from build123d import *

# Parameters (mm, degrees)
CROQUIS1_W              = 4
CROQUIS1_H              = 11
SALIENTE_EXTRUIR1_DEPTH = 100
SALIENTE_EXTRUIR2_DEPTH = 11
REDONDEO1_R             = 10


with BuildPart() as part:
    # Croquis1 → Saliente-Extruir1 (new body)
    with BuildSketch(Plane.XY):
        with Locations((-13, 0)):
            Rectangle(CROQUIS1_W, CROQUIS1_H)
    extrude(amount=-SALIENTE_EXTRUIR1_DEPTH)

    # Croquis3 → Saliente-Extruir2 (add)
    with BuildSketch(Plane.XZ.offset(5.5)):
        Polygon((-15, -100), (-30.130974356, -100), (-15, -76.782527914), align=None)
    extrude(amount=-SALIENTE_EXTRUIR2_DEPTH)

    # Redondeo1
    redondeo1_edges = [part.edges().sort_by_distance(p)[0] for p in [
        (-15, 0, -76.782527914),
    ]]
    fillet(redondeo1_edges, radius=REDONDEO1_R)


solid = part.part
Design review of the part built by this model. Coordinates are the model's own, in mm. A direction names the side the tool comes from. Give positions to 0.01 mm unless a question says otherwise; leave off trailing zeros. Order: outer loops, then holes, each group sorted by start corner. A loop starts at its lowest first (then second) coordinate and runs counter-clockwise, first axis right, second up. Notation, with made-up numbers: (77, -5) - (133, -5) arc R28 cw to (133, 27) - close; hole circle Ø11 at (7, -16). An arc over 180 degrees is marked (long way). Use CSV: the item, a comma, the result in double quotes. Start each with the question number.
Q1. Machinability: for faces 1 (the face through (-15, 0, -36)), 2 (the face through (-20, 0, -100)), which of the approach directions +Z, -Z, +X, -X, +Y, -Y give a long, thin tool a straight path to every point of the face, cutting with its end or side? Answer none if there is none.
Q2. Take a section at C-C (x = -22). State the section outline as (y, z) points, and give its area (3 significant figures).
Q3. For line 1 (X direction, y = 4, z = -39); line 2 (Z direction, x = -28.5, y = 0.5); line 3 (Z direction, x = -24.25, y = 3), list the stretches that pass through material, from the lowest coordinate up.
Q4. Take a section at A-A (y = -0.5). State the section outline as (x, z) points, and give its area (3 significant figures).
Q5. Take a section at B-B (z = -53). State the section outline as (x, y) points, and give its area (3 significant figures).
Q6. For P1, Ø3.5, axis at y = 1.5, z = -55.5, coming from the -X side, flat-tipped, find the tip position at first contact; note if it passes through.
Calculated:
1,face 1,"+Z, -X, +Y, -Y"
1,face 2,"-Z, +X, -X, +Y, -Y"
2,outline,"(-5.5, -100) - (5.5, -100) - (5.5, -87.52) - (-5.5, -87.52) - close"
2,area,"137 mm²"
3,line 1,"x = -15 to -11"
3,line 2,"z = -100 to -97.5"
3,line 3,"z = -100 to -90.98"
4,outline,"(-30.13, -100) - (-11, -100) - (-11, 0) - (-15, 0) - (-15, -73.81) arc R10 cw to (-16.62, -79.27) - close"
4,area,"576 mm²"
5,outline,"(-15, -5.5) - (-11, -5.5) - (-11, 5.5) - (-15, 5.5) - close"
5,area,"44.0 mm²"
6,P1,"stops at x = -15"
